Here's how the part is built. I have some questions about the finished solid (model axes, mm). A direction names the side the tool comes from. Coordinates: 2 decimals unless noted, no trailing zeros. Write each loop counter-clockwise with the first axis right and the second up, starting at its lowest first coordinate (ties: lowest second). Pieces come first, ordered by that corner, then holes. Notation, with made-up numbers: (39, 2) -> (93, 2) arc R17 ccw to (93, 25) -> close; hole circle Ø3 at (83.25, 6.25). An arc over 180 degrees is marked (long way). Put each result on its own line as item: value. Start each with the question number.
Item 1: I need wall thicknesses on line 1 (Z direction, x = -4, y = 10.5); line 2 (Y direction, x = -9, z = 16). Which ranges of each line are inside material? Lowest first, please. Write a range as [from, to].
Item 2: On a 3-axis mill with a long thin cutter (end or side, diameter ignored), from which of +Z, -Z, +X, -X, +Y, -Y can I reach the whole of each face in a straight line? I mean faces 1 (the face through (3.681, 19.076, 14.565)), 2 (the face through (-2, 0, -2)). Say none if no direction works.
Item 3: If we mould it in two halves opening along Z, with no side actions, what happens to faces 3 (the face through (-5, 7, -5)), 4 (the face through (0.59, 3.46, 4.46)), 5 (the face through (8.563, 18.342, -11.701))? For each: released by +Z, released by -Z, zero draft, split by the parting line, or undercut.
Item 4: For pin 1 (1 mm diameter, centred on y = 18.5, z = -0.5, fed in from +X); pin 2 (8 mm diameter, centred on x = -4, z = -1.5, fed in from +Y); pin 3 (6 mm diameter, centred on y = 7, z = -9.5, fed in from -X), each with a flat end and sliding along its axis, tell me the tip position at first contact or that it passes through.
Item 5: I want a section at A-A, the plane y = 2.25. List the corners of the cut face in (x, z) for me, then the cut area to 3 significant figures.
from build123d import *

# Parameters (mm, degrees)
CHAMFER1_SIZE      = 2
CHAMFER1_SIZE2     = 3.464101615
CHAMFER2_SIZE      = 1.5
SKETCH2_W          = 31
SKETCH2_H          = 2
CUT_EXTRUDE1_DEPTH = 15
CIRPATTERN1_COUNT  = 10
CHAMFER3_SIZE      = 5
CHAMFER4_SIZE      = 1


with BuildPart() as part:
    # Sketch1 → Revolve1 (revolve)
    with BuildSketch(Plane.XY):
        Polygon((-2.5, 0), (-2.5, 9), (-4.75, 9), (-4.75, 13), (-14.5, 13), (-14.5, 27), (-20, 27), (-20, 21.3), (-17.5, 21.3), (-17.5, 7), (-6.5, 7), (-6.5, 6), (-4.5, 6), (-4.5, 0), align=None)
    revolve(axis=Axis((0, 0, 0), (0, 1, 0)))

    # Chamfer1
    chamfer1_edges = [part.edges().sort_by_distance(p)[0] for p in [
        (14.5, 27, 0),
    ]]
    chamfer1_side = [part.faces().sort_by_distance(p)[0] for p in [
        (15.065685425, 27, 0),
    ]]
    chamfer(chamfer1_edges, length=CHAMFER1_SIZE, length2=CHAMFER1_SIZE2, reference=chamfer1_side[0])

    # Chamfer2
    chamfer2_edges = [part.edges().sort_by_distance(p)[0] for p in [
        (20, 27, 0),
    ]]
    chamfer(chamfer2_edges, length=CHAMFER2_SIZE)

    # Sketch2 → Cut-Extrude1 (cut, through all)
    with BuildSketch(Plane(origin=(0, 13, 0), x_dir=(1, 0, 0), z_dir=(0, 1, 0))):
        Rectangle(SKETCH2_W, SKETCH2_H)
    cut_extrude1 = extrude(amount=CUT_EXTRUDE1_DEPTH, mode=Mode.SUBTRACT)

    # CirPattern1: Cut-Extrude1 ×10 about axis
    cirpattern1_axis = Axis((0, 0, 0), (0, 1, 0))
    for i in range(1, CIRPATTERN1_COUNT):
        add(cut_extrude1.rotate(cirpattern1_axis, i * 360 / CIRPATTERN1_COUNT), mode=Mode.SUBTRACT)

    # Chamfer3
    chamfer3_edges = [part.edges().sort_by_distance(p)[0] for p in [
        (17.5, 7, 0),
    ]]
    chamfer(chamfer3_edges, length=CHAMFER3_SIZE)

    # Chamfer4
    chamfer4_edges = [part.edges().sort_by_distance(p)[0] for p in [
        (4.5, 0, 0),
    ]]
    chamfer(chamfer4_edges, length=CHAMFER4_SIZE)


solid = part.part
Calculated:
1. line 1: z = [-15.49, -2.56], [2.56, 15.49]
1. line 2: y = [21.3, 27]
2. face 1: +Y
2. face 2: +Z, -Z, +X, -X, -Y
3. face 3: zero draft
3. face 4: split by the parting line
3. face 5: undercut
4. pin 1: stops at x = 17.5
4. pin 2: stops at y = 13
4. pin 3: stops at x = -12.81
5. outline: circle Ø9 at (0, 0); hole circle Ø5 at (0, 0)
5. area: 44.0 mm2
